The model under review builds one solid part; all positions refer to its coordinate system, in mm. A direction names the side the tool comes from. Round coordinates to 2 decimals unless told otherwise and drop trailing zeros. Write each loop counter-clockwise with the first axis right and the second up, starting at its lowest first coordinate (ties: lowest second). Pieces come first, ordered by that corner, then holes. Notation, with made-up numbers: (66.25, 57.25) -> (115.25, 57.25) arc R13 cw to (115.25, 70.25) -> close; hole circle Ø7 at (32, 83.25). An arc over 180 degrees is marked (long way). Answer as a JSON object with one key per item and string values. Group by question number.
1) We need section B-B, the plane x = -1. Write out the cut boundary in (y, z), then the cut area to 3 significant figures.
2) Insertion check: pin 1 Ø4 at (y, z) = (0, 5.5) entering from -X; pin 2 Ø3 at (y, z) = (1, 6) entering from +X; pin 3 Ø1 at (y, z) = (6.5, 1) entering from +X. Each pin has a flat end and moves straight along its axis. Give the tip position at first contact, or say it passes through.
3) Machinability: for faces 1 (the flat face through (1.59, 4.45, 3.94)), 2 (the flat face through (6, 6, -0.8)), 3 (the flat face through (5.106, 5.166, -0.394)), 4 (the flat face through (5.166, 0.894, -0.394)), 5 (the flat face through (0.894, 0.834, -0.394)), which of the approach directions +Z, -Z, +X, -X, +Y, -Y give a long, thin tool a straight path to every point of the face, cutting with its end or side? Answer none if there is none.
4) We need section A-A, the plane y = 6.5. Write out the cut boundary in (x, z).
5) We need section D-D, the plane x = 7.5. Write out the cut boundary in (y, z), then the cut area to 3 significant figures.
6) We need section C-C, the plane z = 1.25. Write out the cut boundary in (x, y).
7) To check wall thickness, follow probe 1 along Z at (x, y) = (1, -1.25); probe 2 along Z at (x, y) = (2.75, 0); probe 3 along X at (y, z) = (4.75, 1.5). State the ranges of each line that lie inside material, in increasing order. Write a range as [from, to].
Autodesk Inventor part; units mm, degrees
ref_plane "YZ Plane" through (0, 0, 0) normal (1, 0, 0) x (0, 1, 0)
ref_plane "XZ Plane" through (0, 0, 0) normal (0, 1, 0) x (-1, 0, 0)
ref_plane "XY Plane" through (0, 0, 0) normal (0, 0, 1) x (1, 0, 0)
sketch "Sketch3" plane through (0, 0, 0) normal (0, 0, 1) x (1, 0, 0)
  line L0 (0, 0) -> (6, 0) construction
  line L1 (6, 0) -> (6, 6) construction
  line L2 (6, 6) -> (0, 6) construction
  line L3 (0, 6) -> (0, 0) construction
  line L4 (0, 0) -> (6, 6) construction
  line L5 (0, 6) -> (6, 0) construction
  line L6 (3, 6) -> (3, 0) construction
  line L7 (6, 3) -> (0, 3) construction
  line L8 (3, 6) -> (6, 3) construction
  line L9 (6, 3) -> (3, 0) construction
  line L10 (3, 0) -> (0, 3) construction
  line L11 (0, 3) -> (3, 6) construction
  line L12 (3, 5.8586) -> (0.1414, 3)
  line L13 (0.1414, 3) -> (3, 0.1414)
  line L14 (3, 0.1414) -> (5.8586, 3)
  line L15 (3, 5.8586) -> (5.8586, 3)
  dimension "d9" = 6
  dimension "d10" = 6
  dimension "d11" = 0.1
  dimension "d12" = 0.1
extrude "Extrusion3" add sketch "Sketch3" along normal blind 8
sketch "Sketch4" plane through (0, 0, 8) normal (0, 0, 1) x (1, 0, 0)
  line L0 (0.1414, 3) -> (5.8586, 3) construction
  line L1 (3, 0.1414) -> (3, 5.8586) construction
  circle A0 centre (3, 3) radius 2.0213
  point P0 (0, 0)
extrude "Extrusion4" add sketch "Sketch4" along normal blind 3
chamfer "Chamfer2" distance 0.5 angle 45 1 edges at (0.9787, 3, 11)
sketch "Sketch5" plane through (0, 0, 0) normal (0, 0, -1) x (-1, 0, 0)
  line L0 (-3, 5.8586) -> (-0.1414, 3)
  line L1 (-5.8586, 3) -> (-3, 5.8586)
  line L2 (-3, 0.1414) -> (-5.8586, 3)
  line L3 (-0.1414, 3) -> (-3, 0.1414)
  line L4 (1.2728, 3) -> (-3, 7.2728)
  line L5 (-3, 7.2728) -> (-7.2728, 3)
  line L6 (-7.2728, 3) -> (-3, -1.2728)
  line L7 (-3, -1.2728) -> (1.2728, 3)
  point P0 (0, 0)
  dimension "d20" = 1
extrude "Extrusion5" add sketch "Sketch5" along normal blind 1 contours L0 L3 L2 L1 | L7 L6 L5 L4
sketch "Sketch6" plane through (0, 0, -1) normal (0, 0, -1) x (-1, 0, 0)
  line L0 (1.2728, 3) -> (-3, 7.2728)
  line L1 (-3, 7.2728) -> (-7.2728, 3)
  line L2 (-7.2728, 3) -> (-3, -1.2728)
  line L3 (-3, -1.2728) -> (1.2728, 3)
  line L4 (-8.684, 8.684) -> (2.4119, 8.684)
  line L5 (2.4119, 8.684) -> (2.4119, -2.7747)
  line L6 (2.4119, -2.7747) -> (-8.684, -2.7747)
  line L7 (-8.684, -2.7747) -> (-8.684, 8.684)
  point P0 (0, 0)
extrude "printing support" add sketch "Sketch6" against normal blind 0.2
equation "\"d12\" = d11"
properties part number "BUTTON"
Here are the results:
{
 "1": {"outline": "(-2.77, -1) -> (8.68, -1) -> (8.68, -0.8) -> (3.27, -0.8) -> (3.27, 0) -> (2.73, 0) -> (2.73, -0.8) -> (-2.77, -0.8) -> close", "area": "2.73 mm^2"},
 "2": {"pin 1": "stops at x = 1.14", "pin 2": "stops at x = 5.36", "pin 3": "passes through"},
 "3": {"face 1": "+Z, -X, +Y", "face 2": "+Z", "face 3": "+Z, +X, +Y", "face 4": "+Z, +X, -Y", "face 5": "+Z, -X, -Y"},
 "4": {"outline": "(-2.41, -1) -> (8.68, -1) -> (8.68, -0.8) -> (3.77, -0.8) -> (3.77, 0) -> (2.23, 0) -> (2.23, -0.8) -> (-2.41, -0.8) -> close"},
 "5": {"outline": "(-2.77, -1) -> (8.68, -1) -> (8.68, -0.8) -> (-2.77, -0.8) -> close", "area": "2.29 mm^2"},
 "6": {"outline": "(0.14, 3) -> (3, 0.14) -> (5.86, 3) -> (3, 5.86) -> close"},
 "7": {"probe 1": "z = [-1, -0.8]", "probe 2": "z = [-1, 0]", "probe 3": "x = [1.89, 4.11]"}
}
